```python
from build123d import *

# Parameters (mm, degrees)
SKETCH_W        = 15
SKETCH_H        = 50
PAD_DEPTH       = 38
SKETCH001_R     = 4.75
POCKET_DEPTH    = 50.001
POCKET001_DEPTH = 15.001
POCKET002_DEPTH = 15.001
SKETCH005_W     = 2.5
SKETCH005_H     = 19.729757
POCKET003_DEPTH = 50.001
SKETCH006_R     = 1.5
POCKET004_DEPTH = 15.001
SKETCH007_R     = 1.875
POCKET005_DEPTH = 7
FILLET_R        = 1


with BuildPart() as part:
    # Sketch → Pad (new body)
    with BuildSketch(Plane.XY):
        Rectangle(SKETCH_W, SKETCH_H)
    extrude(amount=PAD_DEPTH)

    # Sketch001 (on Face3 of Pad) → Pocket (cut, through all)
    with BuildSketch(Plane.XZ.offset(25)):
        with Locations((0, 30)):
            Circle(SKETCH001_R)
    extrude(amount=-POCKET_DEPTH, mode=Mode.SUBTRACT)

    # Sketch003 (on Face5 of Pocket) → Pocket001 (cut, through all)
    with BuildSketch(Plane.YZ.offset(7.5)):
        Polygon((10, 42.759873), (10, 20), (-31.063036, 13.17035), (-31.063036, 49.393513), align=None)
    extrude(amount=-POCKET001_DEPTH, mode=Mode.SUBTRACT)

    # Sketch004 (on Face2 of Pocket001) → Pocket002 (cut, through all)
    with BuildSketch(Plane(origin=(-7.5, 0, 0), x_dir=(0, -1, 0), z_dir=(-1, 0, 0))):
        Polygon((18.707549, -4.016844), (5, 9.690705), (-5, 9.690705), (-5, -5.466326), align=None)
    extrude(amount=-POCKET002_DEPTH, mode=Mode.SUBTRACT)

    # Sketch005 (on Face1 of Pocket002) → Pocket003 (cut, through all)
    with BuildSketch(Plane(origin=(0, 25, 0), x_dir=(-1, 0, 0), z_dir=(0, 1, 0))):
        with Locations((0, 26.377617)):
            Rectangle(SKETCH005_W, SKETCH005_H)
    extrude(amount=-POCKET003_DEPTH, mode=Mode.SUBTRACT)

    # Sketch006 (on Face2 of Pocket003) → Pocket004 (cut, through all)
    with BuildSketch(Plane(origin=(-7.5, 0, 0), x_dir=(0, -1, 0), z_dir=(-1, 0, 0))):
        with Locations((-17.5, 21.974657)):
            Circle(SKETCH006_R)
    extrude(amount=-POCKET004_DEPTH, mode=Mode.SUBTRACT)

    # Sketch007 (on Face2 of Pocket004) → Pocket005 (cut)
    with BuildSketch(Plane(origin=(-7.5, 0, 0), x_dir=(0, -1, 0), z_dir=(-1, 0, 0))):
        with Locations((-17.5, 21.974657)):
            Circle(SKETCH007_R)
    extrude(amount=-POCKET005_DEPTH, mode=Mode.SUBTRACT)

    # Fillet
    fillet_edges = [part.edges().sort_by_distance(p)[0] for p in [
        (-7.5, 17.5, 38),
        (7.5, 17.5, 38),
        (7.5, -7.5, 17.08938),
        (-7.5, -7.5, 17.08938),
    ]]
    fillet(fillet_edges, radius=FILLET_R)


solid = part.part
```
Input: part model. Units: mm. Frame: model coordinates. A direction names the side the tool comes from. Coordinates: 2 decimals unless noted, no trailing zeros. Write each loop counter-clockwise with the first axis right and the second up, starting at its lowest first coordinate (ties: lowest second). Pieces come first, ordered by that corner, then holes. Notation, with made-up numbers: (49, -12) -> (102, -12) arc R15 cw to (102, 12) -> close; hole circle Ø2 at (63, 42.5). An arc over 180 degrees is marked (long way). Write each question's results on one line, items separated by ' | '.
Item 1: Section query C-C on z = 29. Return loops of the section in (x, y).
Conclusion:
outline: (-7.5, 10) -> (-4.64, 10) -> (-4.64, 25) -> (-7.5, 25) -> close; (4.64, 10) -> (7.5, 10) -> (7.5, 25) -> (4.64, 25) -> close
Item 2: Section query B-B on x = -3.25. Return loops of the section in (y, z) (3 decimals).
Conclusion:
outline: (-25, 0) -> (-14.691, 0) -> (-5, 9.691) -> (5, 9.691) -> (5, 0) -> (25, 0) -> (25, 26.536) -> (10, 26.536) -> (10, 20) -> (-25, 14.179) -> close; (10, 33.464) -> (25, 33.464) -> (25, 38) -> (10, 38) -> close; hole circle Ø3.75 at (17.5, 21.975)
Item 3: Section query A-A on y = 17.5. Return loops of the section in (x, z), plus the area to 3 significant figures.
Conclusion:
outline: (-7.5, 0) -> (7.5, 0) -> (7.5, 20.47) -> (1.25, 20.47) -> (1.25, 16.51) -> (-1.25, 16.51) -> (-1.25, 20.1) -> (-7.5, 20.1) -> close; (-7.5, 23.85) -> (-1.25, 23.85) -> (-1.25, 25.42) arc R4.75 cw to (-1.25, 34.58) -> (-1.25, 36.24) -> (1.25, 36.24) -> (1.25, 34.58) arc R4.75 cw to (1.25, 25.42) -> (1.25, 23.47) -> (7.5, 23.47) -> (7.5, 37) arc R1 ccw to (6.5, 38) -> (-6.5, 38) arc R1 ccw to (-7.5, 37) -> close | area: 431 mm^2
Item 4: Section query D-D on x = 3. Return loops of the section in (y, z), plus the area to 3 significant figures.
Conclusion:
outline: (-25, 0) -> (-14.69, 0) -> (-5, 9.69) -> (5, 9.69) -> (5, 0) -> (25, 0) -> (25, 26.32) -> (10, 26.32) -> (10, 20) -> (-25, 14.18) -> close; (10, 33.68) -> (25, 33.68) -> (25, 38) -> (10, 38) -> close; hole circle Ø3 at (17.5, 21.97) | area: 907 mm^2
Item 5: Material intervals for probe 1 along Z at (x, y) = (-6, 17.5); probe 2 along Z at (x, y) = (-4.25, 17.5); probe 3 along Z at (x, y) = (0.25, 14.5), sorted ascending.
Conclusion:
probe 1: z = 0 to 20.1, 23.85 to 38 | probe 2: z = 0 to 20.1, 23.85 to 27.88, 32.12 to 38 | probe 3: z = 0 to 16.51, 36.24 to 38
Item 6: Pin query (flat end, axial travel): pin 1 Ø4.5 at (x, z) = (3.5, 25.5) entering from -Y; pin 2 Ø3.5 at (y, z) = (17.5, 21.97) entering from -X. Return the tip coordinate at first contact, or that it passes through.
Conclusion:
pin 1: stops at y = 10 | pin 2: stops at x = 1.25
Item 7: Set-up query: faces 1 (the flat face through (0, -20, 0)), 2 (the cylindrical face through (-4.419, 19.373, 22.057)), 3 (the flat face through (0, 0, 9.691)), 4 (the flat face through (1.25, 18, 35)). Return all of +Z, -Z, +X, -X, +Y, -Y with unobstructed straight access to the full face (end or side cutting, diameter ignored); none if empty.
Conclusion:
face 1: -Z, +X, -X, +Y, -Y | face 2: -X | face 3: -Z, +X, -X | face 4: +Y, -Y
Item 8: Mould query, pull axis Y, two halves, no side actions, for faces 5 (the cylindrical face through (-7.215, 17.605, 37.699)), 6 (the flat face through (0, -25, 7)), 7 (the flat face through (0, 5, 5)), 8 (the flat face through (-0.1, -9.91, 4.78)). Classes: +Y half, -Y half, draft (parallel to the pull), parting line (faces both ways), or undercut.
Conclusion:
face 5: draft | face 6: -Y half | face 7: undercut | face 8: undercut
